```python
from build123d import *

# Parameters (mm, degrees)
BOSS_EXTRUDE1_DEPTH = 76.2
SKETCH3_OUTSIDE_W   = 23.712
SKETCH3_OUTSIDE_H   = 24.694
SKETCH3_OUTSIDE_R   = 3.175
CUT_EXTRUDE1_DEPTH  = 25.4
SKETCH4_OUTSIDE_W   = 23.712
SKETCH4_OUTSIDE_H   = 24.694
SKETCH4_OUTSIDE_R   = 3.175
CUT_EXTRUDE2_DEPTH  = 15.875


with BuildPart() as part:
    # Sketch2 → Boss-Extrude1 (new body)
    with BuildSketch(Plane.XY):
        Polygon((0, 3.666174209), (-3.175, 1.833087105), (-3.175, -1.833087105), (0, -3.666174209), (3.175, -1.833087105), (3.175, 1.833087105), align=None)
    extrude(amount=BOSS_EXTRUDE1_DEPTH)

    # Sketch3 outside → Cut-Extrude1 (cut)
    with BuildSketch(Plane.XY.offset(76.2)):
        Rectangle(SKETCH3_OUTSIDE_W, SKETCH3_OUTSIDE_H)
        Circle(SKETCH3_OUTSIDE_R, mode=Mode.SUBTRACT)
    extrude(amount=-CUT_EXTRUDE1_DEPTH, mode=Mode.SUBTRACT)

    # Sketch4 outside → Cut-Extrude2 (cut)
    with BuildSketch(Plane(origin=(0, 0, 0), x_dir=(-1, 0, 0), z_dir=(0, 0, -1))):
        Rectangle(SKETCH4_OUTSIDE_W, SKETCH4_OUTSIDE_H)
        Circle(SKETCH4_OUTSIDE_R, mode=Mode.SUBTRACT)
    extrude(amount=-CUT_EXTRUDE2_DEPTH, mode=Mode.SUBTRACT)


solid = part.part
```
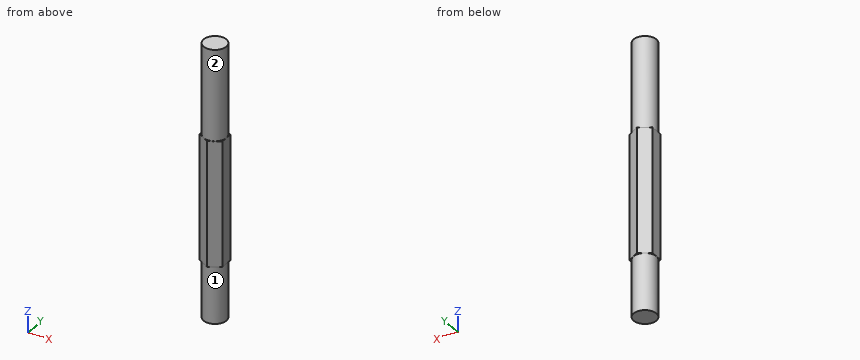
Geometry check sheet. Reference: the model listing, model coordinates, mm. Face numbers are marked on the shaded views. A direction names the side the tool comes from. Coordinates: 2 decimals unless noted, no trailing zeros. Order: outer loops, then holes, each group sorted by start corner. A loop starts at its lowest first (then second) coordinate and runs counter-clockwise, first axis right, second up. Notation, with made-up numbers: (88, 75) - (145, 75) arc R24 cw to (145, 94) - close; hole circle Ø8 at (38, 41.5). An arc over 180 degrees is marked (long way). Answer as a JSON object with one key per item and string values. Group by question number.
Item 1: Sectioned sample at C-C, the plane z = 63. Record the cut outline in (x, y) (3 decimals).
Item 2: Sectioned sample at B-B, the plane x = -2.25. Record the cut outline in (y, z) (3 decimals).
Item 3: Sectioned sample at A-A, the plane z = 42. Record the cut outline in (x, y) (3 decimals), and give its area (3 significant figures).
Item 4: Tool access check on the marked faces 1 and 2. Record the directions out of +Z, -Z, +X, -X, +Y, -Y that give a thin tool (end or side, any length) a straight path to the whole face; none if there is none.
Item 5: Scan lines: probe 1 along Y at (x, z) = (0.25, 9); probe 2 along Z at (x, y) = (2.75, -2) (3 decimals); probe 3 along X at (y, z) = (-2.75, 66). Record each from-to range of solid material in increasing order.
Item 6: Depth check by flat-ended pin: pin 1 Ø0.5 at (x, y) = (-2.5, 1.5) entering from -Z; pin 2 Ø1.5 at (y, z) = (-2.5, 55) entering from -X; pin 3 Ø2 at (y, z) = (2, 12.5) entering from +X. Enter the tip coordinate at first touch or a pass-through.
Resolved:
{
 "1": {"outline": "circle Ø6.35 at (0, 0)"},
 "2": {"outline": "(-2.367, 15.875) - (-2.24, 15.875) - (-2.24, 0) - (2.24, 0) - (2.24, 15.875) - (2.367, 15.875) - (2.367, 50.8) - (2.24, 50.8) - (2.24, 76.2) - (-2.24, 76.2) - (-2.24, 50.8) - (-2.367, 50.8) - close"},
 "3": {"outline": "(-3.175, -1.833) - (0, -3.666) - (3.175, -1.833) - (3.175, 1.833) - (0, 3.666) - (-3.175, 1.833) - close", "area": "34.9 mm^2"},
 "4": {"face 1": "-Z", "face 2": "+Z"},
 "5": {"probe 1": "-3.17 to 3.17", "probe 2": "15.875 to 50.8", "probe 3": "-1.59 to 1.59"},
 "6": {"pin 1": "z = 0", "pin 2": "x = -2.65", "pin 3": "x = 3.01"}
}
